```python
from build123d import *

# Parameters (mm, degrees)
SKETCH1_W = 47.908763192
SKETCH1_H = 51.416423574
SKETCH3_R = 9.608888213


with BuildPart() as part:
    # Sketch1 → Revolve1 (revolve)
    with BuildSketch(Plane.XY):
        with Locations((-52.129799597, 25.708211787)):
            Rectangle(SKETCH1_W, SKETCH1_H)
    revolve(axis=Axis((0, 0, 0), (0, 1, 0)))

    # Sketch3 → Cut-Revolve1 (revolve, cut)
    with BuildSketch(Plane.XY):
        with Locations((-76.084181193, 25.708211787)):
            Circle(SKETCH3_R)
    revolve(axis=Axis((0, 0, 0), (0, 1, 0)), mode=Mode.SUBTRACT)


solid = part.part
```
Part model, mm, in its own coordinate system. Round coordinates to 2 decimals unless told otherwise and drop trailing zeros. Loops run counter-clockwise (first coordinate to the right, second up) from the corner with the lowest first, then second, coordinate; pieces in that order, holes last. Notation, with made-up numbers: (50, 85.5) -> (95, 85.5) arc R26 ccw to (95, 111.5) -> close; hole circle Ø7 at (14, -15.5). An arc over 180 degrees is marked (long way). Use CSV: the item, a comma, the result in double quotes. Start each with the question number.
1) Cut at A-A, the plane z = 0. Write the cut outline in (x, y).
2) Pull direction Z, two halves, no side cores. Call faces 1 (the flat face through (1, 51.416, -33)), 2 (the cylindrical face through (-72.57, 43.48, 22.85)), 3 (the cylindrical face through (20.77, 26.07, 19.04)): +Z half, -Z half, draft (parallel to the pull), parting line (faces both ways), or undercut.
3) Cut at B-B, the plane x = 0. Write the cut outline in (y, z).
4) Cut at D-D, the plane y = 32. Write the cut outline in (x, z), plus the area to 3 significant figures.
5) Cut at C-C, the plane y = 5.5. Write the cut outline in (x, z).
6) Drop flat-ended pins along their axis: P1, Ø12, axis at x = 24.5, y = 26.5, coming from the +Z side; P2, Ø12, axis at x = -28.5, y = 11.5, coming from the +Z side; P3, Ø2, axis at y = 6.5, z = 34.5, coming from the +X side. Give the stop position or say it passes through.
7) Wall check: L1, parallel to Z at x = 0, y = 11; L2, parallel to X at y = 38.5, z = 1; L3, parallel to Z at x = -4, y = 43. Give the ranges that are in metal, low to high. Write a range as [from, to].
Determined:
1,outline,"(-76.08, 0) -> (-28.18, 0) -> (-28.18, 51.42) -> (-76.08, 51.42) -> (-76.08, 35.32) arc R9.61 cw to (-76.08, 16.1) -> close; (28.18, 0) -> (76.08, 0) -> (76.08, 16.1) arc R9.61 cw to (76.08, 35.32) -> (76.08, 51.42) -> (28.18, 51.42) -> close"
2,face 1,"draft"
2,face 2,"parting line"
2,face 3,"undercut"
3,outline,"(0, -76.08) -> (16.1, -76.08) arc R9.61 cw to (35.32, -76.08) -> (51.42, -76.08) -> (51.42, -28.18) -> (0, -28.18) -> close; (0, 28.18) -> (51.42, 28.18) -> (51.42, 76.08) -> (35.32, 76.08) arc R9.61 cw to (16.1, 76.08) -> (0, 76.08) -> close"
4,outline,"circle Ø137.64 at (0, 0); hole circle Ø56.35 at (0, 0)"
4,area,"12,400 mm2"
5,outline,"circle Ø152.17 at (0, 0); hole circle Ø56.35 at (0, 0)"
6,P1,"stops at z = 65.19"
6,P2,"stops at z = 72.68"
6,P3,"stops at x = 68.31"
7,L1,"z = [-76.08, -28.18], [28.18, 76.08]"
7,L2,"x = [-76.08, -28.16], [28.16, 76.08]"
7,L3,"z = [-75.98, -27.89], [27.89, 75.98]"
